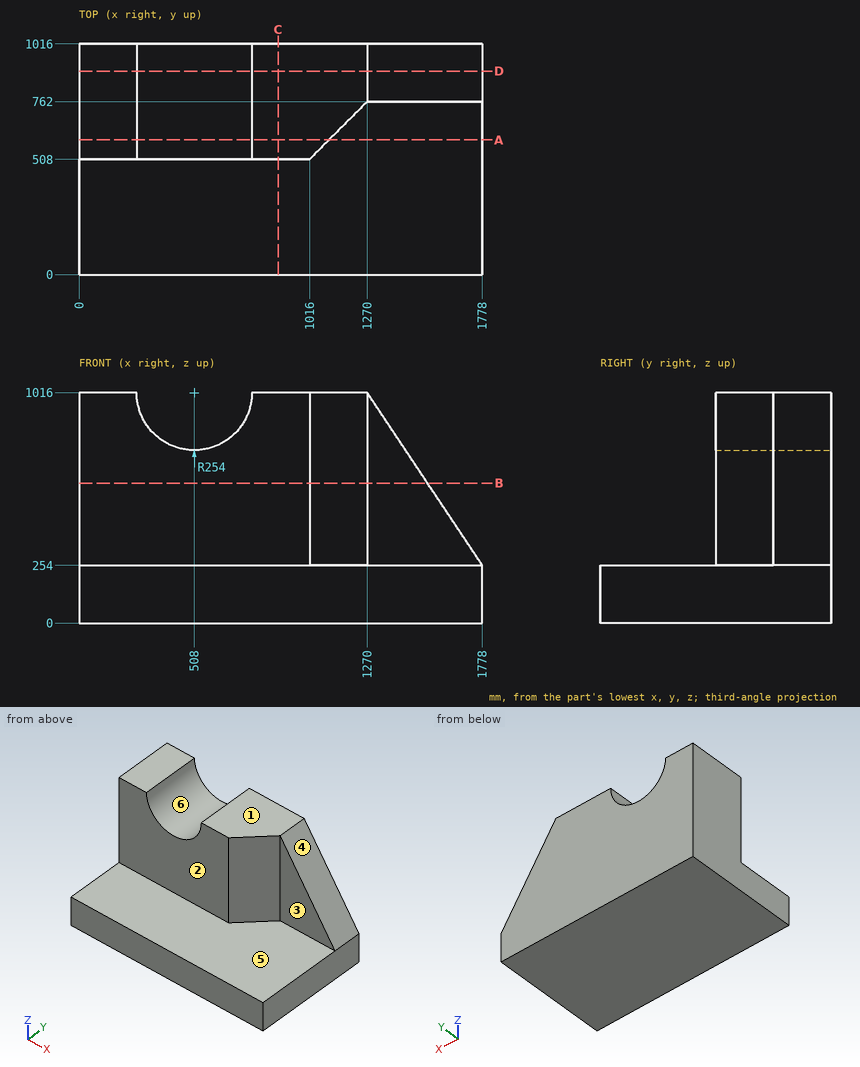
Study the drawing (mm; zero at the part's minimum x, y, z) and answer. A direction names the side the tool comes from. Give positions to 0.01 mm unless a question says otherwise; leave off trailing zeros. Order: outer loops, then holes, each group sorted by start corner. A loop starts at its lowest first (then second) coordinate and runs counter-clockwise, first axis right, second up. Notation, with made-up numbers: (51.25, -5.75) - (94.25, -5.75) arc R13 cw to (94.25, 11.25) - close; hole circle Ø4 at (11, -4). An arc over 180 degrees is marked (long way). Use one line per item in the form item = value. Start each with the question number.
(1) A cutting plane is placed at D-D, the plane y = 896.5. Write down the section's boundary in (x, z), then the cut area to 3 significant figures.
(2) Consider line 1 (Y direction, x = 1276.5, z = 260.5); line 2 (Z direction, x = 1052.5, y = 386.5); line 3 (Y direction, x = 690, z = 358). Determine where each line is inside the solid, lowest interval first. Write a range as from..to.
(3) A cutting plane is placed at B-B, the plane z = 617. Write down the section's boundary in (x, y), then the cut area to 3 significant figures.
(4) For the marked faces 1, 2 and 3, determine the directions among +Z, -Z, +X, -X, +Y, -Y from which every point of the face is accessible in a straight line to the end or side of a thin tool.
(5) Flat-ended cylindrical pins translate along their axes: pin 1 Ø10 at (y, z) = (887, 869) entering from +X; pin 2 Ø1 at (x, y) = (557, 295.5) entering from +Z; pin 3 Ø4 at (y, z) = (653, 436) entering from +X. Find the tip coordinate at first contact, or state that the pin passes through.
(6) The mould has two halves that part along X. Classify the marked faces 4, 5 and 6: released by +X, released by -X, zero draft, split by the parting line, or undercut.
(7) A cutting plane is placed at A-A, the plane y = 594. Write down the section's boundary in (x, z).
(8) A cutting plane is placed at C-C, the plane x = 877. Write down the section's boundary in (y, z).
Ans:
q1.outline = (0, 0) - (1778, 0) - (1778, 254) - (1270, 1016) - (762, 1016) arc R254 cw to (254, 1016) - (0, 1016) - close
q1.area = 1,510,000 mm^2
q2.line_1 = 762..1016
q2.line_2 = 0..254
q2.line_3 = 508..1016
q3.outline = (0, 508) - (1016, 508) - (1270, 762) - (1536, 762) - (1536, 1016) - (0, 1016) - close
q3.area = 680,000 mm^2
q4.face_1 = +Z, +X, -X, +Y, -Y
q4.face_2 = +Z, +X, -X, -Y
q4.face_3 = +Z, +X, -Y
q5.pin_1 = 1371.33
q5.pin_2 = 254
q5.pin_3 = 1163
q6.face_4 = released by +X
q6.face_5 = zero draft
q6.face_6 = undercut
q7.outline = (0, 0) - (1778, 0) - (1778, 254) - (1102, 254) - (1102, 1016) - (762, 1016) arc R254 cw to (254, 1016) - (0, 1016) - close
q8.outline = (0, 0) - (1016, 0) - (1016, 1016) - (508, 1016) - (508, 254) - (0, 254) - close
